```python
from build123d import *

# Parameters (mm, degrees)
F0_W     = 3.175
F0_H     = 3.175
F0_W_2   = 47.625
F0_H_2   = 47.625
F1_DEPTH = 1524


with BuildPart() as f1:
    # F0 (on Front) → F1 (new body)
    with BuildSketch(Plane.XZ):
        with Locations((1.5875, 1.5875)):
            Rectangle(F0_W, F0_H)
        with Locations((26.9875, 1.5875)):
            Rectangle(F0_W_2, F0_H)
        with Locations((1.5875, 26.9875)):
            Rectangle(F0_W, F0_H_2)
    extrude(amount=-F1_DEPTH)


solid = f1.part
```
Verification items for the finished model (mm, model axes). A direction names the side the tool comes from. Give positions to 0.01 mm unless a question says otherwise; leave off trailing zeros. Order: outer loops, then holes, each group sorted by start corner. A loop starts at its lowest first (then second) coordinate and runs counter-clockwise, first axis right, second up. Notation, with made-up numbers: M -35,-30 L -13,-30 A22 ccw -13,-18 Z; hole C 16.25,75 d10. An arc over 180 degrees is marked long. Answer in a Markdown table with one row per item. Add a question column.
Item 1: Section check C-C, the plane x = 20. Enter the section's corners in (y, z) (3 decimals), and give its area (3 significant figures).
Item 2: Scan line: probe 1 along X at (y, z) = (1277, 12.5) (3 decimals). Record every from-to range of solid material in increasing order. Write a range as from..to.
Item 3: Tool access check on faces 1 (the flat face through (3, 0, 14)), 2 (the flat face through (27, 751, 3.175)). Record the directions out of +Z, -Z, +X, -X, +Y, -Y that give a thin tool (end or side, any length) a straight path to the whole face; none if there is none.
Item 4: Section check A-A, the plane y = 759.5. Enter the section's corners in (x, z) (3 decimals).
Item 5: Gauge pin test, flat ends, axial feed: pin 1 (12 mm diameter, centred on x = 17, y = 1370, fed in from +Z) (3 decimals); pin 2 (14.5 mm diameter, centred on y = 593.5, z = 24.5, fed in from +X) (3 decimals). Record the tip position at first contact, or that the pin passes through.
Item 6: Section check B-B, the plane z = 40.5. Enter the section's corners in (x, y) (3 decimals), and give its area (3 significant figures).
Filled sheet:
| question | item | result |
|---|---|---|
| 1 | outline | M 0,0 L 1524,0 L 1524,3.175 L 0,3.175 Z |
| 1 | area | 4,840 mm^2 |
| 2 | probe 1 | x = 0..3.175 |
| 3 | face 1 | +Z, -Z, +X, -X, -Y |
| 3 | face 2 | +Z, +X, +Y, -Y |
| 4 | outline | M 0,0 L 50.8,0 L 50.8,3.175 L 3.175,3.175 L 3.175,50.8 L 0,50.8 Z |
| 5 | pin 1 | stops at z = 3.175 |
| 5 | pin 2 | stops at x = 3.175 |
| 6 | outline | M 0,0 L 3.175,0 L 3.175,1524 L 0,1524 Z |
| 6 | area | 4,840 mm^2 |
